The model under review builds one solid part; all positions refer to its coordinate system, in mm. A direction names the side the tool comes from. Coordinates: 2 decimals unless noted, no trailing zeros. Write each loop counter-clockwise with the first axis right and the second up, starting at its lowest first coordinate (ties: lowest second). Pieces come first, ordered by that corner, then holes. Notation, with made-up numbers: (53.5, -24) -> (86.5, -24) arc R23 ccw to (86.5, 14) -> close; hole circle Ø5 at (46, 77). An arc over 180 degrees is marked (long way). Write each question's results on one line, items separated by ' | '.
```python
from build123d import *

# Parameters (mm, degrees)
F0_W           = 380
F0_H           = 330
F1_DEPTH       = 10
F2_W           = 320.3
F2_H           = 294.3
F3_DEPTH       = 203
F4_W           = 47.5
F4_H           = 42
F4_R           = 13
F5_DEPTH       = 30.5
F7_D           = 6
F7_DEPTH       = 10
F8_D           = 5.5
F8_DEPTH       = 10
F8_CSINK_D     = 10
F8_CSINK_ANGLE = 90


with BuildPart() as f1:
    # F0 (on Top) → F1 (new body)
    with BuildSketch(Plane.XY):
        Rectangle(F0_W, F0_H)
    extrude(amount=F1_DEPTH)

    # F2 (on face) → F3 (join)
    with BuildSketch(Plane(origin=(0, 0, 0), x_dir=(1, 0, 0), z_dir=(0, 0, -1))):
        Rectangle(F2_W, F2_H)
    extrude(amount=F3_DEPTH)

    # F4 (on face) → F5 (join)
    with BuildSketch(Plane.XY.offset(10)):
        with Locations((-43.5, -46.5)):
            Rectangle(F4_W, F4_H)
        with Locations((-43.5, -46.5)):
            Circle(F4_R, mode=Mode.SUBTRACT)
    extrude(amount=F5_DEPTH)

    # F7
    with Locations(Plane.XY.offset(10)):
        with Locations((-182, 135), (-182, -135), (182, 135), (182, -135), (10, -157), (-10, 157)):
            Hole(F7_D / 2, depth=F7_DEPTH)

    # F8
    with Locations(Plane.XY.offset(10)):
        with Locations((-182, 145), (182, 145), (-182, -145), (182, -145), (0, -157), (0, 157)):
            CounterSinkHole(F8_D / 2, F8_CSINK_D / 2, depth=F8_DEPTH, counter_sink_angle=F8_CSINK_ANGLE)


solid = f1.part
```
Q1. Add section D-D (y = -46.5). Write out the cut boundary in (x, z), plus the area to 3 significant figures.
Solution:
outline: (-190, 0) -> (-160.15, 0) -> (-160.15, -203) -> (160.15, -203) -> (160.15, 0) -> (190, 0) -> (190, 10) -> (-19.75, 10) -> (-19.75, 40.5) -> (-30.5, 40.5) -> (-30.5, 10) -> (-56.5, 10) -> (-56.5, 40.5) -> (-67.25, 40.5) -> (-67.25, 10) -> (-190, 10) -> close | area: 69,500 mm²
Q2. Clearance check with flat-ended pins moving along their axes: P1, Ø3, axis at x = -44, y = 6.5, coming from the +Z side; P2, Ø9, axis at y = -38.5, z = 18, coming from the -X side; P3, Ø6, axis at x = 48, z = -147, coming from the +Y side. State where each tip first meets the part, or that it passes through.
Solution:
P1: z = 10 | P2: x = -67.25 | P3: y = 147.15
Q3. Add section A-A (y = 99). Write out the cut boundary in (x, z).
Solution:
outline: (-190, 0) -> (-160.15, 0) -> (-160.15, -203) -> (160.15, -203) -> (160.15, 0) -> (190, 0) -> (190, 10) -> (-190, 10) -> close
Q4. Machinability: for faces 1 (the cylindrical face through (-53.08, -37.71, 25.04)), 2 (the flat face through (-19.75, -47, 25)), 3 (the flat face through (-2, -147.15, -100)), 4 (the flat face through (-67.25, -47, 25)), which of the approach directions +Z, -Z, +X, -X, +Y, -Y give a long, thin tool a straight path to every point of the face, cutting with its end or side? Answer none if there is none.
Solution:
face 1: +Z | face 2: +Z, +X, +Y, -Y | face 3: -Z, +X, -X, -Y | face 4: +Z, -X, +Y, -Y
Q5. Add section C-C (z = -91). Write out the cut boundary in (x, y).
Solution:
outline: (-160.15, -147.15) -> (160.15, -147.15) -> (160.15, 147.15) -> (-160.15, 147.15) -> close
Q6. Add section B-B (x = -74). Write out the cut boundary in (y, z), plus the area to 3 significant figures.
Solution:
outline: (-165, 0) -> (-147.15, 0) -> (-147.15, -203) -> (147.15, -203) -> (147.15, 0) -> (165, 0) -> (165, 10) -> (-165, 10) -> close | area: 63,000 mm²
Q7. For line 1 (X direction, y = -135, z = 9.5); line 2 (X direction, y = 145, z = 3.25); line 3 (Y direction, x = 182, z = 4.75), list the stretches that pass through material, from the lowest coordinate up. Write a range as from..to.
Solution:
line 1: -190..-185, -179..179, 185..190 | line 2: -190..-184.75, -179.25..179.25, 184.75..190 | line 3: -165..-147.75, -142.25..-138, -132..132, 138..142.25, 147.75..165
Q8. Draft analysis for pull direction Y (two halves, no side actions). For faces 5 (the flat face through (-160.15, 2, -100)), 6 (the flat face through (-3, -165, 5)), 7 (the conical face through (180.46, 147.41, 7.86)), state which applies: pulls with the +Y half, pulls with the -Y half, needs draft (parallel to the pull), parting line crosses it, or undercut.
Solution:
face 5: needs draft | face 6: pulls with the -Y half | face 7: undercut
